Verification items for this drawing (mm, ordinates from the low corner). A direction names the side the tool comes from. Round coordinates to 2 decimals unless told otherwise and drop trailing zeros. Loops run counter-clockwise (first coordinate to the right, second up) from the corner with the lowest first, then second, coordinate; pieces in that order, holes last. Notation, with made-up numbers: M 5,-3.5 L 63,-3.5 A32 ccw 63,24.5 Z; hole C 46,12.5 d2. An arc over 180 degrees is marked long. Write item = value, one per line. Start each with the question number.
(1) Cross-section at A-A on y = 25.4. Record the boundary of the cut face in (x, z) (3 decimals).
(2) Cross-section at B-B on z = 34. Record the boundary of the cut face in (x, y) (3 decimals), plus the area to 3 significant figures.
(3) Cross-section at C-C on y = 18.5. Record the boundary of the cut face in (x, z).
(4) Go/stop test with flat-tipped pins: P1, Ø17, axis at x = 61.5, y = 27, coming from the +Z side; P2, Ø20.5, axis at y = 23.5, z = 43.5, coming from the +X side; P3, Ø5, axis at y = 25.4, z = 38.1, coming from the -X side. Record where each tip stops, or that it passes through.
(5) Scan lines: L1, parallel to X at y = 25.4, z = 47; L2, parallel to Z at x = 28.5, y = 25.4 (3 decimals); L3, parallel to Y at x = 16, z = 38. Record each from-to range of solid material in increasing order. Write a range as from..to.
(6) Set-up check for the marked faces 1 and 2: record each of +Z, -Z, +X, -X, +Y, -Y from which the full face is reachable in a straight line by a thin tool's end or side.
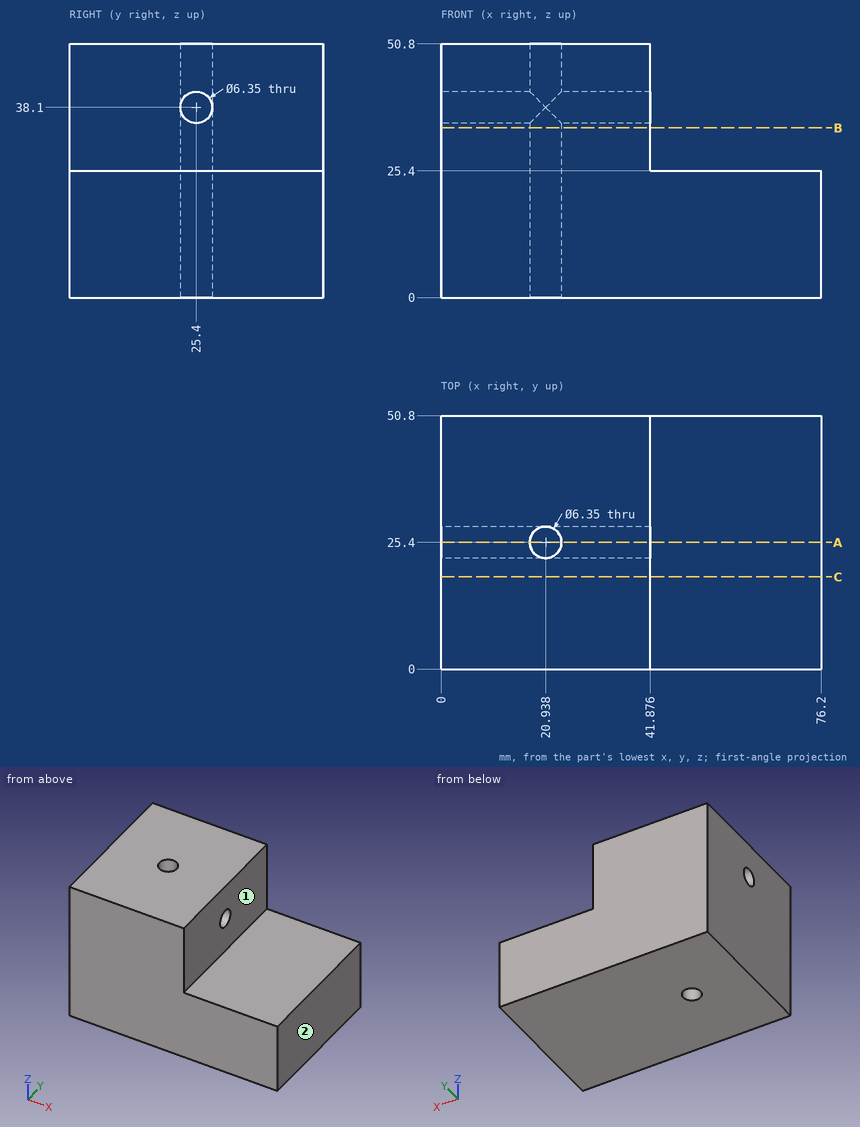
Result:
q1.outline = M 0,0 L 17.763,0 L 17.763,34.925 L 0,34.925 Z; M 0,41.275 L 17.763,41.275 L 17.763,50.8 L 0,50.8 Z; M 24.113,0 L 76.2,0 L 76.2,25.4 L 41.876,25.4 L 41.876,34.925 L 24.113,34.925 Z; M 24.113,41.275 L 41.876,41.275 L 41.876,50.8 L 24.113,50.8 Z
q2.outline = M 0,0 L 41.876,0 L 41.876,50.8 L 0,50.8 Z; hole C 20.938,25.4 d6.35
q2.area = 2,100 mm^2
q3.outline = M 0,0 L 76.2,0 L 76.2,25.4 L 41.88,25.4 L 41.88,50.8 L 0,50.8 Z
q4.P1 = 25.4
q4.P2 = 41.88
q4.P3 = through
q5.L1 = 0..17.76, 24.11..41.88
q5.L2 = 0..34.925, 41.275..50.8
q5.L3 = 0..22.23, 28.57..50.8
q6.face_1 = +Z, +X, +Y, -Y
q6.face_2 = +Z, -Z, +X, +Y, -Y
